Check sheet for the modelled part. Datum: model origin and axes. Units: mm. A direction names the side the tool comes from. Round coordinates to 2 decimals unless told otherwise and drop trailing zeros. Write each loop counter-clockwise with the first axis right and the second up, starting at its lowest first coordinate (ties: lowest second). Pieces come first, ordered by that corner, then holes. Notation, with made-up numbers: (46.5, 3) - (74.5, 3) arc R23 ccw to (74.5, 25) - close; hole circle Ø3 at (-36, 11.25). An arc over 180 degrees is marked (long way). Use one line per item in the form item = value. Start each with the question number.
1) Scan lines: probe 1 along X at (y, z) = (2.75, -4.75); probe 2 along Z at (x, y) = (-16, -3); probe 3 along Y at (x, z) = (15.15, 0). Record each from-to range of solid material in increasing order.
2) Section check B-B (x = -12.5). Record the boundary of the cut face in (y, z).
3) Gauge pin test, flat ends, axial feed: P1, Ø3, axis at x = 13, y = -3.5, coming from the -Z side; P2, Ø1, axis at x = 2, y = 4, coming from the +Z side; P3, Ø0.6, axis at x = -0.5, y = 7.5, coming from the +Z side. Record the tip position at first contact, or that the pin passes through.
4) Section check C-C (x = 9.5). Record the boundary of the cut face in (y, z), then the cut area to 3 significant figures.
5) Draft check along X on faces 4 (the face through (13.5, -1, -1)), 5 (the face through (-13.5, 2, -5)), 6 (the face through (-18.74, 4.05, -2.58)). Enter one of: +X half, -X half, draft (parallel to the pull), parting line (faces both ways), or undercut.
6) Set-up check for faces 1 (the face through (18.74, -4.05, -2.58)), 2 (the face through (10, 7, 0)), 3 (the face through (13.5, 2, -5)): record each of +Z, -Z, +X, -X, +Y, -Y from which the full face is reachable in a straight line by a thin tool's end or side.
7) Section check A-A (x = -19). Record the boundary of the cut face in (y, z), then the cut area to 3 significant figures.
Autodesk Inventor part; units mm, degrees
ref_plane "Work Plane1" through (18, 0, 0) normal (1, 0, 0) x (0, 0, -1)
ref_plane "YZ Plane" through (0, 0, 0) normal (1, 0, 0) x (0, 1, 0)
ref_plane "XZ Plane" through (0, 0, 0) normal (0, 1, 0) x (-1, 0, 0)
sketch "Sketch1" plane through (0, 0, 0) normal (1, 0, 0) x (0, 1, 0)
  circle A0 centre (0, 0) radius 6.5
  dimension "d0" = 13
extrude "Extrusion1" add sketch "Sketch1" along normal mid plane 27
sketch "Sketch2" plane through (13.5, 0, 0) normal (1, 0, 0) x (0, 0, -1)
  circle A0 centre (0, 0) radius 5
  dimension "d3" = 10
extrude "Extrusion2" add sketch "Sketch2" along normal blind 12
ref_plane "Work Plane1" through (18, 0, 0) normal (1, 0, 0) x (0, 0, -1)
sketch "Sketch3" plane through (18, 0, 0) normal (1, 0, 0) x (0, 0, -1)
  circle A0 centre (0, 0) radius 4.8
  circle A1 centre (0, 0) radius 5
  dimension "d8" = 9.6
extrude "Extrusion3" cut sketch "Sketch3" along normal blind 1.5
mirror "Mirror1" about plane through (0, 0, 0) normal (1, 0, 0) of "Extrusion2", "Extrusion3"
sketch "Sketch4" plane through (0, 0, 0) normal (0, 1, 0) x (-1, 0, 0)
  line L0 (7.5, 0) -> (-7.5, 0) construction
  line L1 (7.5, -2.5) -> (-7.5, -2.5)
  line L2 (-7.5, 2.5) -> (7.5, 2.5)
  arc A0 (7.5, -2.5) -> (7.5, 2.5) centre (7.5, 0) ccw
  arc A1 (-7.5, 2.5) -> (-7.5, -2.5) centre (-7.5, 0) ccw
  point P0 (0, 0)
  point P1 (0, 0)
  point P2 (10, 0)
  point P3 (-10, 0)
  dimension "d11" = 5
  dimension "d12" = 20
  dimension "d13" = 10
  dimension "d14" = 0
extrude "Extrusion4" add sketch "Sketch4" along normal blind 8
fillet "Fillet2" radius 1 1 edges at (-25.5, 0, 5)
sketch "Sketch6" plane through (25.5, 0, 0) normal (1, 0, 0) x (0, 0, -1)
  circle A0 centre (0, 0) radius 5
extrude "Extrusion6" add sketch "Sketch6" along normal blind 2
sketch "Sketch8" plane through (27.5, 0, 0) normal (1, 0, 0) x (0, 0, -1)
  circle A0 centre (0, 0) radius 3
  line L0 (1.0445, 2.8123) -> (-2.8123, -1.0445)
  line L1 (-2.1213, -2.1213) -> (4.9809, 4.9809)
  line L2 (9.1, 0) -> (-9.1, 0)
  point P0 (-0.8839, 0.8839)
  dimension "d30" = 6
  dimension "d31" = 45
  dimension "d32" = 1.25
extrude "Extrusion8" cut sketch "Sketch8" against normal blind 10.6 contours L0 L2 L1 A0 | L1 L2 A0 | L0 A0 L1 L2 | L2 L1 A0
sketch "Sketch9" plane through (27.5, 0, 0) normal (1, 0, 0) x (0, 0, -1)
  arc A0 (-2.8123, -1.0445) -> (1.0445, 2.8123) centre (0, 0) ccw
  line L0 (-2.8123, -1.0445) -> (1.0445, 2.8123)
  circle A1 centre (0, 0) radius 5
extrude "Extrusion9" cut sketch "Sketch9" against normal blind 4.6
sketch "Sketch10" plane through (22.9, 0, 0) normal (1, 0, 0) x (0, 0, -1)
  circle A0 centre (0, 0) radius 5
  line L0 (1.0445, 2.8123) -> (-2.8123, -1.0445)
  arc A1 (-2.8123, -1.0445) -> (1.0445, 2.8123) centre (0, 0) ccw
extrude "Extrusion10" cut sketch "Sketch10" against normal blind 1.4
sketch "Sketch11" plane through (16.9, 0, 0) normal (1, 0, 0) x (0, 0, -1)
  line L0 (-2.8123, -1.0445) -> (1.0445, 2.8123)
  arc A0 (-2.8123, -1.0445) -> (1.0445, 2.8123) centre (0, 0) ccw
extrude "Extrusion11" cut sketch "Sketch11" against normal up to surface (3.4 mm away)
properties part number "Shaft between link2 and 3"
Results are:
q1.probe_1 = -13.5 to 13.5
q1.probe_2 = -4 to 4
q1.probe_3 = -5 to -3, 1.77 to 5
q2.outline = circle Ø13 at (0, 0)
q3.P1 = -6.18
q3.P2 = 5.48
q3.P3 = 2.5
q4.outline = (6.32, -1.5) - (8, -1.5) - (8, 1.5) - (6.32, 1.5) arc R6.5 ccw (long way) to start
q4.area = 137 mm²
q5.face_4 = +X half
q5.face_5 = -X half
q5.face_6 = undercut
q6.face_1 = none
q6.face_2 = +X, +Y
q6.face_3 = +X
q7.outline = circle Ø9.6 at (0, 0)
q7.area = 72.4 mm²
